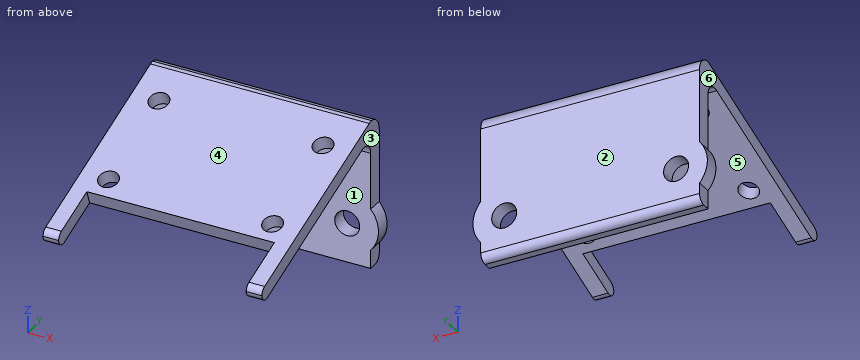
from build123d import *

# Parameters (mm, degrees)
SZKIC1_W                    = 28
SZKIC1_H                    = 19
DODANIE_WYCI_GNI_CIE1_DEPTH = 2
SZKIC2_R                    = 1.6
WYTNIJ_WYCI_GNI_CIE1_DEPTH  = 18.036725037
SZKIC7_R                    = 4
SZKIC7_R_2                  = 1.6
DODANIE_WYCI_GNI_CIE3_DEPTH = 2
DODANIE_WYCI_GNI_CIE2_DEPTH = 28
SZKIC4_R                    = 1.25
WYTNIJ_WYCI_GNI_CIE2_DEPTH  = 1.879385242
WYTNIJ_WYCI_GNI_CIE4_DEPTH  = 33.297362502
ZAOKR_GLENIE1_R             = 2
ZAOKR_GLENIE2_R             = 1.5
ZAOKR_GLENIE3_R             = 1
ZAOKR_GLENIE4_R             = 1


with BuildPart() as part:
    # Szkic1 → Dodanie-wyciągnięcie1 (new body)
    with BuildSketch(Plane(origin=(0, 0, 0), x_dir=(1, 0, 0), z_dir=(0, 1, 0))):
        Rectangle(SZKIC1_W, SZKIC1_H)
    extrude(amount=DODANIE_WYCI_GNI_CIE1_DEPTH)

    # Szkic2 → Wytnij-wyciągnięcie1 (cut, through all)
    with BuildSketch(Plane(origin=(0, 2, 0), x_dir=(1, 0, 0), z_dir=(0, 1, 0))):
        with Locations(Location((11, 4.5, 0), (0, 0, 270))):
            Circle(SZKIC2_R)
        with Locations(Location((-11, 4.5, 0), (0, 0, 90))):
            Circle(SZKIC2_R)
    extrude(amount=-WYTNIJ_WYCI_GNI_CIE1_DEPTH, mode=Mode.SUBTRACT)

    # Szkic7 → Dodanie-wyciągnięcie3 (add)
    with BuildSketch(Plane(origin=(0, 2, 0), x_dir=(1, 0, 0), z_dir=(0, 1, 0))):
        with Locations((11, 4.5)):
            Circle(SZKIC7_R)
        with Locations(Location((11, 4.5, 0), (0, 0, 270))):
            Circle(SZKIC7_R_2, mode=Mode.SUBTRACT)
    dodanie_wyci_gni_cie3 = extrude(amount=-DODANIE_WYCI_GNI_CIE3_DEPTH)

    # Lustro1: Dodanie-wyciągnięcie3 across plane
    add(dodanie_wyci_gni_cie3.mirror(Plane(origin=(0, 0, 0), x_dir=(0, 0, 1), z_dir=(1, 0, 0))))

    # Szkic3 → Dodanie-wyciągnięcie2 (add)
    with BuildSketch(Plane(origin=(14, 0, 0), x_dir=(0, 0, -1), z_dir=(1, 0, 0))):
        Polygon((-9.5, 0), (-0.26545613, -25.371700761), (1.73454387, -25.371700761), (-7.5, 0), align=None)
    extrude(amount=-DODANIE_WYCI_GNI_CIE2_DEPTH)

    # Szkic4 → Wytnij-wyciągnięcie2 (cut)
    with BuildSketch(Plane(origin=(0, -3.053241146, 8.388711105), x_dir=(1, 0, 0), z_dir=(0, -0.3420201433256705, 0.9396926207859079))):
        with Locations(Location((-10.5, -1.787484051, 0), (0, 0, 270))):
            Circle(SZKIC4_R)
        with Locations(Location((-10.5, -14.287484051, 0), (0, 0, 270))):
            Circle(SZKIC4_R)
        with Locations(Location((10.5, -14.287484051, 0), (0, 0, 90))):
            Circle(SZKIC4_R)
        with Locations(Location((10.5, -1.787484051, 0), (0, 0, 90))):
            Circle(SZKIC4_R)
    extrude(amount=-WYTNIJ_WYCI_GNI_CIE2_DEPTH, mode=Mode.SUBTRACT)

    # Szkic6 → Wytnij-wyciągnięcie4 (cut, through all)
    with BuildSketch(Plane(origin=(0, -3.053241146, 8.388711105), x_dir=(1, 0, 0), z_dir=(0, -0.3420201433256704, 0.9396926207859078))):
        Polygon((-12, -23.750808638), (-12, -16.750808638), (12, -16.750808638), (12, -23.750808638), (12, -25.909421261), (-12, -25.909421261), align=None)
    extrude(amount=-WYTNIJ_WYCI_GNI_CIE4_DEPTH, mode=Mode.SUBTRACT)

    # Zaokrąglenie1
    # the kernel refuses this fillet: 2 mm, written as the material it takes off along each edge
    with BuildSketch(Plane(origin=(-19, 2, 9.5), x_dir=(0, -1, 0), z_dir=(1, 0, 0))) as zaokr_glenie1_piece_1:
        with BuildLine():
            CenterArc((ZAOKR_GLENIE1_R, ZAOKR_GLENIE1_R), ZAOKR_GLENIE1_R, 180, 90)
            Line((0, ZAOKR_GLENIE1_R), (0, 0))
            Line((0, 0), (ZAOKR_GLENIE1_R, 0))
        make_face()
    extrude(amount=38, mode=Mode.SUBTRACT)
    with BuildSketch(Plane(origin=(-14.881634904, 0, 9.5), x_dir=(0, 1, 0), z_dir=(1, 0, 0))) as zaokr_glenie1_piece_2:
        with BuildLine():
            CenterArc((ZAOKR_GLENIE1_R * 0.176326980708, -ZAOKR_GLENIE1_R), ZAOKR_GLENIE1_R, 90, 20)
            Line((-ZAOKR_GLENIE1_R * 0.165693162617, -ZAOKR_GLENIE1_R * 0.0603073792141), (0, 0))
            Line((0, 0), (ZAOKR_GLENIE1_R * 0.176326980708, 0))
        make_face()
    extrude(amount=29.763269807, mode=Mode.SUBTRACT)

    # Zaokrąglenie2
    zaokr_glenie2_edges = [part.edges().sort_by_distance(p)[0] for p in [
        (0, 0, 7.5),
    ]]
    fillet(zaokr_glenie2_edges, radius=ZAOKR_GLENIE2_R)

    # Zaokrąglenie3
    # the kernel refuses this fillet: 1 mm, written as the material it takes off along each edge
    with BuildSketch(Plane(origin=(17.570370017, -25.371700761, -1.73454387), x_dir=(0, 0.9396926207859079, 0.34202014332567016), z_dir=(-1, 0, 0)), Plane(origin=(-8.429629983, -25.371700761, -1.73454387), x_dir=(0, 0.9396926207859079, 0.34202014332567016), z_dir=(-1, 0, 0))) as zaokr_glenie3_piece_1:
        with BuildLine():
            CenterArc((ZAOKR_GLENIE3_R * 1.42814800674, -ZAOKR_GLENIE3_R), ZAOKR_GLENIE3_R, 90, 110)
            Line((ZAOKR_GLENIE3_R * 0.488455385956, -ZAOKR_GLENIE3_R * 1.34202014333), (0, 0))
            Line((0, 0), (ZAOKR_GLENIE3_R * 1.42814800674, 0))
        make_face()
    extrude(amount=9.140740034, mode=Mode.SUBTRACT)
    with BuildSketch(Plane(origin=(-10.249481154, -25.371700761, 0.26545613), x_dir=(0, 0.9396926207859077, 0.34202014332567093), z_dir=(-1, 0, 0))) as zaokr_glenie3_piece_2:
        with BuildLine():
            CenterArc((ZAOKR_GLENIE3_R * 0.70020753821, ZAOKR_GLENIE3_R), ZAOKR_GLENIE3_R, 200, 70)
            Line((-ZAOKR_GLENIE3_R * 0.239485082576, ZAOKR_GLENIE3_R * 0.657979856674), (0, 0))
            Line((0, 0), (ZAOKR_GLENIE3_R * 0.70020753821, 0))
        make_face()
    extrude(amount=5.501037691, mode=Mode.SUBTRACT)
    with BuildSketch(Plane(origin=(15.750518846, -25.371700761, 0.26545613), x_dir=(0, 0, -1), z_dir=(-1, 0, 0))) as zaokr_glenie3_piece_3:
        with BuildLine():
            CenterArc((ZAOKR_GLENIE3_R * 0.70020753821, -ZAOKR_GLENIE3_R), ZAOKR_GLENIE3_R, 90, 70)
            Line((-ZAOKR_GLENIE3_R * 0.239485082576, -ZAOKR_GLENIE3_R * 0.657979856674), (0, 0))
            Line((0, 0), (ZAOKR_GLENIE3_R * 0.70020753821, 0))
        make_face()
    extrude(amount=5.501037691, mode=Mode.SUBTRACT)

    # Zaokrąglenie4
    zaokr_glenie4_edges = [part.edges().sort_by_distance(p)[0] for p in [
        (0, 2, -9.5),
    ]]
    fillet(zaokr_glenie4_edges, radius=ZAOKR_GLENIE4_R)


solid = part.part
The model under review builds one solid part; all positions refer to its coordinate system, in mm. Face numbers are marked on the shaded views. A direction names the side the tool comes from. Give positions to 0.01 mm unless a question says otherwise; leave off trailing zeros. Loops run counter-clockwise (first coordinate to the right, second up) from the corner with the lowest first, then second, coordinate; pieces in that order, holes last. Notation, with made-up numbers: (62.5, -0.5) -> (93.5, -0.5) arc R21 cw to (93.5, 6.5) -> close; hole circle Ø3 at (89.25, 48.5). An arc over 180 degrees is marked (long way). Put each result on its own line as item: value. Start each with the question number.
1. We need section A-A on z = -4.5. State the section outline as (x, y) points, then the cut area to 3 significant figures.
2. For the marked faces 4, 5 and 6, list the 3-axis set-ups (+Z, -Z, +X, -X, +Y, -Y) from which the entire face can be reached by the end or side of a thin tool; tool diameter is ignored.
3. We need section C-C on x = 7.75. State the section outline as (y, z) points, then the cut area to 3 significant figures.
4. Clearance check with flat-ended pins moving along their axes: P1, Ø2, axis at x = -11.5, y = -17, coming from the -Z side; P2, Ø1, axis at x = 11.5, y = -9, coming from the +Z side; P3, Ø9, axis at y = -6, z = 2, coming from the -X side; P4, Ø1.9, axis at x = 11, z = -4.5, coming from the -Y side. State where each tip first meets the part, or that it passes through.
5. Mouldability with a two-part tool opening along Y and no side actions: class the marked faces 1, 2 and 3 as released by +Y, released by -Y, zero draft, split by the parting line, or undercut.
6. We need section B-B on z = 4.5. State the section outline as (x, y) points, then the cut area to 3 significant figures.
7. Wall thickness on probe 1 along X at (y, z) = (1.35, -4.5); probe 2 along Y at (x, z) = (13.25, -4); probe 3 along Z at (x, y) = (-11, 0.7): over which ranges is each line inside the solid? List them lowest first.
8. We need section D-D on x = 11. State the section outline as (y, z) points, then the cut area to 3 significant figures.
Determined:
1. outline: (-15, 0) -> (-12.6, 0) -> (-12.6, 2) -> (-15, 2) -> close; (-9.4, 0) -> (9.4, 0) -> (9.4, 2) -> (-9.4, 2) -> close; (12.6, 0) -> (15, 0) -> (15, 2) -> (12.6, 2) -> close
1. area: 47.2 mm^2
2. face 4: +Z, +X, -X, -Y
2. face 5: -Z, +X, -X
2. face 6: +Z, -X, +Y, -Y
3. outline: (-18.79, 2.66) -> (-18.15, 0.89) -> (-2.01, 6.77) arc R1.5 cw to (0, 5.36) -> (0, -9.5) -> (1, -9.5) arc R1 ccw to (2, -8.5) -> (2, 7.5) arc R2 ccw to (0.18, 9.49) arc R2 ccw to (-0.33, 9.38) -> close
3. area: 74.9 mm^2
4. P1: z = 0.95
4. P2: z = 6.41
4. P3: x = -14
4. P4: through
5. face 1: undercut
5. face 2: released by +Y
5. face 3: zero draft
6. outline: (-14, -13.74) -> (14, -13.74) -> (14, -8.24) -> (-14, -8.24) -> close; (-14, 0) -> (14, 0) -> (14, 2) -> (-14, 2) -> close
6. area: 210 mm^2
7. probe 1: -15 to -12.6, -9.4 to 9.4, 12.6 to 15
7. probe 2: 0 to 2
7. probe 3: -9.5 to -6.1, -2.9 to 9.37
8. outline: (-18.79, 2.66) -> (-18.15, 0.89) -> (-16.91, 1.34) -> (-17.56, 3.11) -> close; (-15.4, 3.89) -> (-14.76, 2.13) -> (-5.17, 5.62) -> (-5.81, 7.39) -> close; (-3.66, 8.17) -> (-3.01, 6.4) -> (-2.01, 6.77) arc R1.5 cw to (0, 5.36) -> (0, -2.9) -> (2, -2.9) -> (2, 7.5) arc R2 ccw to (0.18, 9.49) arc R2 ccw to (-0.33, 9.38) -> close; (0, -9.5) -> (1, -9.5) arc R1 ccw to (2, -8.5) -> (2, -6.1) -> (0, -6.1) -> close
8. area: 59.9 mm^2
